Verification items for the finished model (mm, model axes). Coordinates: 2 decimals unless noted, no trailing zeros. Loops run counter-clockwise (first coordinate to the right, second up) from the corner with the lowest first, then second, coordinate; pieces in that order, holes last. Notation, with made-up numbers: (-20.5, 74.25) - (5.5, 74.25) arc R21 ccw to (5.5, 81.25) - close; hole circle Ø10 at (11, -35). An arc over 180 degrees is marked (long way). One line per item, written item: value. Start each with the question number.
(1) Gauge pin test, flat ends, axial feed: P1, Ø1, axis at y = 699, z = 2, coming from the +X side; P2, Ø1.6, axis at x = 16, z = 1, coming from the -Y side; P3, Ø1, axis at y = 678.5, z = 1, coming from the +X side. Record the tip position at first contact, or that the pin passes through.
(2) Section check D-D (x = 83.5). Record the boundary of the cut face in (y, z) (3 decimals), plus the area to 3 significant figures.
(3) Section check C-C (y = 676). Record the boundary of the cut face in (x, z) (3 decimals).
(4) Section check A-A (x = 38.1). Record the boundary of the cut face in (y, z) (3 decimals).
(5) Section check B-B (z = 0.75). Record the boundary of the cut face in (x, y) (3 decimals), plus the area to 3 significant figures.
(6) Thickness scan on probe 1 along X at (y, z) = (723, 2.85); probe 2 along Y at (x, z) = (21, 1.4); probe 3 along Y at (x, z) = (12.7, 2.2). Record the ranges inside material, lowest first. Write a range as [from, to].
```python
from build123d import *

# Parameters (mm, degrees)
SKETCH1_R           = 2.5019
BOSS_EXTRUDE1_DEPTH = 3.175
FILLET1_R           = 3.175


with BuildPart() as part:
    # Sketch1 → Boss-Extrude1 (new body)
    with BuildSketch(Plane.XY):
        Polygon((50.8, 696.232068306), (72.893120941, 668.941577789), (92.634850884, 684.923570745), (52.636012774, 734.332068306), (0, 734.332068306), (0, 708.932068306), (40.518666443, 708.932068306), align=None)
        with Locations((66.781992956, 696.67430421)):
            Circle(SKETCH1_R, mode=Mode.SUBTRACT)
        with Locations((74.772989434, 686.803439238)):
            Circle(SKETCH1_R, mode=Mode.SUBTRACT)
        with Locations((12.7, 721.632068306)):
            Circle(SKETCH1_R, mode=Mode.SUBTRACT)
        with Locations((38.1, 721.632068306)):
            Circle(SKETCH1_R, mode=Mode.SUBTRACT)
    extrude(amount=BOSS_EXTRUDE1_DEPTH)

    # Fillet1
    fillet1_edges = [part.edges().sort_by_distance(p)[0] for p in [
        (52.636012774, 734.332068306, 1.5875),
        (92.634850884, 684.923570745, 1.5875),
        (72.893120941, 668.941577789, 1.5875),
        (40.518666443, 708.932068306, 1.5875),
        (0, 708.932068306, 1.5875),
        (0, 734.332068306, 1.5875),
    ]]
    fillet(fillet1_edges, radius=FILLET1_R)


solid = part.part
```
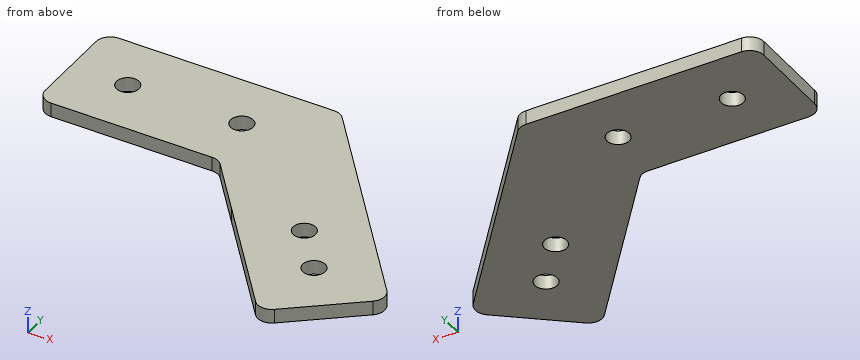
Responses:
1. P1: stops at x = 81.64
1. P2: stops at y = 708.93
1. P3: stops at x = 85.32
2. outline: (677.528, 0) - (696.207, 0) - (696.207, 3.175) - (677.528, 3.175) - close
2. area: 59.3 mm²
3. outline: (67.179, 0) - (81.612, 0) - (81.612, 3.175) - (67.179, 3.175) - close
4. outline: (708.932, 0) - (719.13, 0) - (719.13, 3.175) - (708.932, 3.175) - close; (724.134, 0) - (734.332, 0) - (734.332, 3.175) - (724.134, 3.175) - close
5. outline: (0, 712.107) arc R3.175 ccw to (3.175, 708.932) - (39.004, 708.932) arc R3.175 cw to (41.472, 707.755) - (70.895, 671.409) arc R3.175 ccw to (75.361, 670.939) - (90.167, 682.926) arc R3.175 ccw to (90.637, 687.391) - (53.589, 733.155) arc R3.175 ccw to (51.121, 734.332) - (3.175, 734.332) arc R3.175 ccw to (0, 731.157) - close; hole circle Ø5.004 at (12.7, 721.632); hole circle Ø5.004 at (38.1, 721.632); hole circle Ø5.004 at (66.782, 696.674); hole circle Ø5.004 at (74.773, 686.803)
5. area: 2,560 mm²
6. probe 1: x = [0, 10.61], [14.79, 36.01], [40.19, 61.81]
6. probe 2: y = [708.93, 734.33]
6. probe 3: y = [708.93, 719.13], [724.13, 734.33]
